Autodesk Inventor part; units mm, degrees
ref_plane "YZ Plane" through (0, 0, 0) normal (1, 0, 0) x (0, 1, 0)
ref_plane "XZ Plane" through (0, 0, 0) normal (0, 1, 0) x (-1, 0, 0)
ref_plane "XY Plane" through (0, 0, 0) normal (0, 0, 1) x (1, 0, 0)
sketch "Sketch1" plane through (0, 0, 0) normal (0, 0, 1) x (1, 0, 0)
  line L0 (0, 0) -> (14, 0)
  line L1 (14, 0) -> (14, 9)
  line L2 (14, 9) -> (0, 9)
  line L3 (0, 9) -> (0, 0)
  dimension "d0" = 14
  dimension "d1" = 9
extrude "Extrusion1" add sketch "Sketch1" along normal blind 3
sketch "Sketch2" plane through (0, 0, 3) normal (0, 0, 1) x (1, 0, 0)
  line L0 (1, 1) -> (13, 1)
  line L1 (13, 1) -> (13, 8)
  line L2 (13, 8) -> (1, 8)
  line L3 (1, 8) -> (1, 1)
  dimension "d4" = 12
  dimension "d5" = 7
extrude "Extrusion2" cut sketch "Sketch2" against normal through all
sketch "Sketch3" plane through (0, 9, 0) normal (0, 1, 0) x (1, 0, 0)
  line L0 (0, -3) -> (14, -3)
  line L1 (14, 0) -> (0, 0)
  line L2 (0, 0) -> (0, -3)
  line L3 (6, -3) -> (10, -3)
  line L4 (10, -3) -> (10, 0)
  line L5 (10, 0) -> (6, 0)
  line L6 (6, 0) -> (6, -3)
  dimension "d13" = 4
  dimension "d14" = 6
extrude "Extrusion3" add sketch "Sketch3" along normal blind 4 contours L6 L1 L4 L0
sketch "Sketch5" plane through (0, 0, 3) normal (0, 0, 1) x (1, 0, 0)
  line L0 (13, 8) -> (13, 1)
  line L1 (13, 1) -> (1, 1)
  line L2 (1, 1) -> (1, 8)
  line L3 (1, 8) -> (13, 8)
  line L4 (0.5, 8.5) -> (0.5, 0.5)
  line L5 (0.5, 0.5) -> (13.5, 0.5)
  line L6 (13.5, 0.5) -> (13.5, 8.5)
  line L7 (13.5, 8.5) -> (0.5, 8.5)
  point P0 (14, 1)
  dimension "d17" = 0.5
extrude "Extrusion4" cut sketch "Sketch5" against normal blind 1.1
sketch "Sketch6" plane through (0, 0, 3) normal (0, 0, 1) x (1, 0, 0)
  line L0 (10, 9) -> (10, 13)
  line L1 (10, 13) -> (6, 13)
  line L2 (6, 9) -> (6, 13)
  line L3 (6, 11) -> (10, 11) construction
  line L4 (8, 13) -> (8, 9) construction
  point P0 (8, 11.005)
hole "Hole1" at (8, 11.005, 3) direction (0, 0, -1) diameter 1.524 end through all
thread "Thread1"
sketch "Sketch7" plane through (0, 0, 0) normal (0, -1, 0) x (1, 0, 0)
  line L0 (0, 0) -> (0, 3)
  line L1 (0, 0) -> (14, 0)
  line L2 (7, 0) -> (9, 0)
  line L3 (9, 0) -> (9, 1)
  line L4 (9, 1) -> (7, 1)
  line L5 (7, 1) -> (7, 0)
  dimension "d29" = 2
  dimension "d30" = 1
  dimension "d31" = 7
extrude "Extrusion5" add sketch "Sketch7" along normal blind 1
fillet "Fillet1" radius 0.5 18 edges at (0.5, 0.5, 2.45) (1, 1, 0.95) (1, 8, 0.95) (0.5, 8.5, 2.45) (13, 8, 0.95) (13.5, 8.5, 2.45) (13, 1, 0.95) (13.5, 0.5, 2.45) (14, 0, 1.5) (9, 0, 0.5) (0, 0, 1.5) (7, 0, 0.5) (0, 9, 1.5) (6, 9, 1.5) (6, 13, 1.5) (10, 13, 1.5) (10, 9, 1.5) (14, 9, 1.5)
properties part number "base"
Work out the finished part from the listing and answer in its coordinate system (mm). A direction names the side the tool comes from. Coordinates: 2 decimals unless noted, no trailing zeros. Loops run counter-clockwise (first coordinate to the right, second up) from the corner with the lowest first, then second, coordinate; pieces in that order, holes last. Notation, with made-up numbers: M -31,72.5 L -3,72.5 A34 ccw -3,106.5 Z; hole C 62.5,43 d10. An arc over 180 degrees is marked long. Answer in a Markdown table with one row per item. Add a question column.
1. Find section B-B, the plane y = 4.25. Write down the section's boundary in (x, z), then the cut area to 3 significant figures.
2. Consider L1, parallel to Y at x = 8, z = 1.8; L2, parallel to Y at x = 8, z = 2.1; L3, parallel to X at y = 2, z = 1. Determine where each line is inside the solid, lowest interval first.
3. The mould has two halves that part along Y. Classify faces 1 (the flat face through (6.9, 0, 1.5)), 2 (the flat face through (7, 8, 1)), 3 (the flat face through (0, 5, 1)), 4 (the flat face through (0.5, 4.5, 2.5)): pulls with the +Y half, pulls with the -Y half, needs draft (parallel to the pull), parting line crosses it, or undercut.
4. Flat-ended cylindrical pins translate along their axes: P1, Ø0.9, axis at y = 11.5, z = 2, coming from the +X side; P2, Ø1, axis at x = 4.5, z = 0.5, coming from the -Y side; P3, Ø0.8, axis at x = 7.5, y = -0.5, coming from the +Z side. Find the tip coordinate at first contact, or state that the pin passes through.
5. Find section D-D, the plane z = 0.3. State how many separate pieces and enclosed holes the cut face has, then the cut area to 3 significant figures.
6. A tool of negligible diameter and unlimited length cuts with its end or side. For faces 5 (the flat face through (7.1, 8.5, 2.5)), 6 (the flat face through (1, 5, 1)), 7 (the flat face through (12, 9, 1)), 8 (the flat face through (8, -0.5, 1)), from which of +Z, -Z, +X, -X, +Y, -Y can it reach the whole face along a straight path? Write none if from no direction.
7. Find section C-C, the plane x = 8. Write down the section's boundary in (y, z).
8. Find section A-A, the plane z = 1.2. Write down the section's boundary in (x, y) (3 decimals), then the cut area to 3 significant figures.
Reported:
| question | item | result |
|---|---|---|
| 1 | outline | M 0,0 L 1,0 L 1,1.9 L 0.5,1.9 L 0.5,3 L 0,3 Z; M 13,0 L 14,0 L 14,3 L 13.5,3 L 13.5,1.9 L 13,1.9 Z |
| 1 | area | 4.90 mm^2 |
| 2 | L1 | y = 0 to 1, 8 to 10.24, 11.77 to 13 |
| 2 | L2 | y = 0 to 0.5, 8.5 to 10.24, 11.77 to 13 |
| 2 | L3 | x = 0 to 1, 13 to 14 |
| 3 | face 1 | pulls with the -Y half |
| 3 | face 2 | undercut |
| 3 | face 3 | needs draft |
| 3 | face 4 | undercut |
| 4 | P1 | stops at x = 10 |
| 4 | P2 | stops at y = 0 |
| 4 | P3 | stops at z = 1 |
| 5 | separate pieces | 1 |
| 5 | enclosed holes | 2 |
| 5 | area | 58.3 mm^2 |
| 6 | face 5 | +Z |
| 6 | face 6 | +Z, -Z |
| 6 | face 7 | +Z, -Z, +X, +Y |
| 6 | face 8 | +Z, +X, -X, -Y |
| 7 | outline | M -1,0 L 1,0 L 1,1.9 L 0.5,1.9 L 0.5,3 L 0,3 L 0,1 L -1,1 Z; M 8,0 L 10.24,0 L 10.24,3 L 8.5,3 L 8.5,1.9 L 8,1.9 Z; M 11.77,0 L 13,0 L 13,3 L 11.77,3 Z |
| 8 | outline | M 0,0.5 A0.5 ccw 0.5,0 L 13.5,0 A0.5 ccw 14,0.5 L 14,8.5 A0.5 ccw 13.5,9 L 10.5,9 A0.5 cw 10,9.5 L 10,12.5 A0.5 ccw 9.5,13 L 6.5,13 A0.5 ccw 6,12.5 L 6,9.5 A0.5 cw 5.5,9 L 0.5,9 A0.5 ccw 0,8.5 Z; hole M 1,1.5 A0.5 ccw 1.5,1 L 12.5,1 A0.5 ccw 13,1.5 L 13,7.5 A0.5 ccw 12.5,8 L 1.5,8 A0.5 ccw 1,7.5 Z; hole C 8,11.005 d1.524 |
| 8 | area | 56.2 mm^2 |
